CAD build for the part. Positions are in the model's coordinates, mm. Face numbers are marked on the shaded views. A direction names the side the tool comes from. Round coordinates to 2 decimals unless told otherwise and drop trailing zeros. Loops run counter-clockwise (first coordinate to the right, second up) from the corner with the lowest first, then second, coordinate; pieces in that order, holes last.
from build123d import *

# Parameters (mm, degrees)
BOSS_EXTRUDE1_DEPTH = 50
BOSS_EXTRUDE2_DEPTH = 5
SKETCH3_R           = 50
BOSS_EXTRUDE3_DEPTH = 5
FILLET1_R           = 5
BOSS_EXTRUDE4_START = 3
SKETCH5_R           = 50
BOSS_EXTRUDE4_DEPTH = 3
SKETCH5_3_R         = 4
CUT_EXTRUDE1_DEPTH  = 10


with BuildPart() as part:
    # Sketch1 → Boss-Extrude1 (new body)
    with BuildSketch(Plane(origin=(0, 0, 0), x_dir=(1, 0, 0), z_dir=(0, 1, 0))):
        Polygon((-14.60696181, 25.3), (-29.213923621, 0), (-14.60696181, -25.3), (14.60696181, -25.3), (29.213923621, 0), (14.60696181, 25.3), align=None)
        Polygon((-11.720210465, -20.3), (11.720210465, -20.3), (23.440420929, 0), (11.720210465, 20.3), (-11.720210465, 20.3), (-23.440420929, 0), align=None, mode=Mode.SUBTRACT)
    extrude(amount=BOSS_EXTRUDE1_DEPTH)

    # Sketch2 → Boss-Extrude2 (add)
    with BuildSketch(Plane(origin=(0, 50, 0), x_dir=(1, 0, 0), z_dir=(0, 1, 0))):
        Polygon((-14.60696181, 25.3), (-29.213923621, 0), (-14.60696181, -25.3), (14.60696181, -25.3), (29.213923621, 0), (14.60696181, 25.3), align=None)
    extrude(amount=BOSS_EXTRUDE2_DEPTH)

    # Sketch3 → Boss-Extrude3 (add)
    # profile 1 of 2: a face of its own
    with BuildSketch(Plane.XZ):
        with Locations(Location((0, 0, 0), (0, 0, 270))):
            Circle(SKETCH3_R)
        Polygon((-29.213923621, 0), (-14.60696181, -25.3), (14.60696181, -25.3), (29.213923621, 0), (14.60696181, 25.3), (-14.60696181, 25.3), align=None, mode=Mode.SUBTRACT)
    # profile 2 of 2: a face of its own
    with BuildSketch(Plane.XZ):
        Polygon((-14.60696181, 25.3), (-29.213923621, 0), (-14.60696181, -25.3), (14.60696181, -25.3), (29.213923621, 0), (14.60696181, 25.3), align=None)
        Polygon((-23.440420929, 0), (-11.720210465, 20.3), (11.720210465, 20.3), (23.440420929, 0), (11.720210465, -20.3), (-11.720210465, -20.3), align=None, mode=Mode.SUBTRACT)
    extrude(amount=-BOSS_EXTRUDE3_DEPTH)

    # Fillet1
    fillet1_edges = [part.edges().sort_by_distance(p)[0] for p in [
        (0, 5, -25.3),
        (-21.910442716, 5, 12.65),
        (-21.910442716, 5, -12.65),
        (21.910442716, 5, -12.65),
        (21.910442716, 5, 12.65),
        (0, 5, 25.3),
    ]]
    fillet(fillet1_edges, radius=FILLET1_R)

    # Sketch5 → Boss-Extrude4 (add)
    with BuildSketch(Plane.XZ.offset(BOSS_EXTRUDE4_START)):
        with Locations(Location((0, 0, 0), (0, 0, 270))):
            Circle(SKETCH5_R)
        Polygon((-4.252388339, -34.798222074), (3.484105268, -34.798222074), (7.352352072, -41.498222074), (3.484105268, -48.198222074), (-4.252388339, -48.198222074), (-8.120635142, -41.498222074), align=None, mode=Mode.SUBTRACT)
        Polygon((-32.262338492, -13.716434709), (-28.394091688, -20.416434709), (-32.262338492, -27.116434709), (-39.998832099, -27.116434709), (-43.867078902, -20.416434709), (-39.998832099, -13.716434709), align=None, mode=Mode.SUBTRACT)
        Polygon((28.009950153, -21.081787365), (31.878196957, -14.381787365), (39.614690564, -14.381787365), (43.482937367, -21.081787365), (39.614690564, -27.781787365), (31.878196957, -27.781787365), align=None, mode=Mode.SUBTRACT)
        Polygon((-28.009950153, 21.081787365), (-31.878196957, 14.381787365), (-39.614690564, 14.381787365), (-43.482937367, 21.081787365), (-39.614690564, 27.781787365), (-31.878196957, 27.781787365), align=None, mode=Mode.SUBTRACT)
        Polygon((-11.720210465, -20.3), (-23.440420929, 0), (-11.720210465, 20.3), (11.720210465, 20.3), (23.440420929, 0), (11.720210465, -20.3), align=None, mode=Mode.SUBTRACT)
        Polygon((32.262338492, 13.716434709), (28.394091688, 20.416434709), (32.262338492, 27.116434709), (39.998832099, 27.116434709), (43.867078902, 20.416434709), (39.998832099, 13.716434709), align=None, mode=Mode.SUBTRACT)
        Polygon((4.252388339, 34.798222074), (-3.484105268, 34.798222074), (-7.352352072, 41.498222074), (-3.484105268, 48.198222074), (4.252388339, 48.198222074), (8.120635142, 41.498222074), align=None, mode=Mode.SUBTRACT)
    extrude(amount=-BOSS_EXTRUDE4_DEPTH)

    # Sketch5_3 → Cut-Extrude1 (cut)
    with BuildSketch(Plane.XZ):
        with Locations(Location((0.384141535, 41.498222074, 0), (0, 0, 270))):
            Circle(SKETCH5_3_R)
        with Locations(Location((36.130585295, 20.416434709, 0), (0, 0, 270))):
            Circle(SKETCH5_3_R)
        with Locations(Location((35.74644376, -21.081787365, 0), (0, 0, 270))):
            Circle(SKETCH5_3_R)
        with Locations(Location((-0.384141535, -41.498222074, 0), (0, 0, 270))):
            Circle(SKETCH5_3_R)
        with Locations(Location((-36.130585295, -20.416434709, 0), (0, 0, 270))):
            Circle(SKETCH5_3_R)
        with Locations(Location((-35.74644376, 21.081787365, 0), (0, 0, 270))):
            Circle(SKETCH5_3_R)
    extrude(amount=-CUT_EXTRUDE1_DEPTH, mode=Mode.SUBTRACT)


solid = part.part
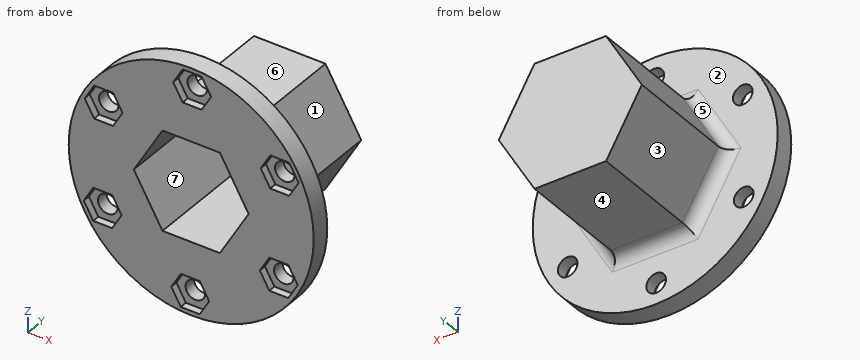
Item 1: Cut at A-A (y = 12). List the corners of the cut face in (x, z).
Verdict:
outline: (-29.21, 0) - (-14.61, -25.3) - (14.61, -25.3) - (29.21, 0) - (14.61, 25.3) - (-14.61, 25.3) - close; hole (-23.44, 0) - (-11.72, -20.3) - (11.72, -20.3) - (23.44, 0) - (11.72, 20.3) - (-11.72, 20.3) - close
Item 2: Wall check: L1, parallel to Z at x = -10.5, y = 43.5; L2, parallel to X at y = 1.5, z = -19; L3, parallel to Y at x = 10.5, z = 10. Give the ranges that are in metal, low to high.
Verdict:
L1: z = -25.3 to -20.3, 20.3 to 25.3
L2: x = -46.25 to -39.87, -32.39 to -12.47, 12.47 to 32.33, 39.16 to 46.25
L3: y = 50 to 55
Item 3: Flat gauge pins, fed straight in: P1, Ø6, axis at y = 47.5, z = 20, coming from the +X side; P2, Ø3.5, axis at x = -36.5, y = -2, coming from the +Z side; P3, Ø2.5, axis at x = 37, y = -1.5, coming from the -Z side; P4, Ø10.5, axis at x = -35, z = 18.5, coming from the -Y side. Where does each tip first touch, or does it go through?
Verdict:
P1: stops at x = 19.4
P2: stops at z = 35.95
P3: stops at z = -34.96
P4: stops at y = -3
Item 4: 3-axis set-ups, long thin cutter, end or side, ignore diameter. For the marked faces 1, 2, 3 and 4: which of +Z, -Z, +X, -X, +Y, -Y reach the whole face in a straight line?
Verdict:
face 1: +Z, +X, +Y
face 2: +Y
face 3: -Z, -X, +Y
face 4: -Z, +X, -X, +Y
Item 5: Mould opens along X. For the marked faces 5, 6 and 7 say: released by +X, released by -X, zero draft, split by the parting line, or undercut.
Verdict:
face 5: released by -X
face 6: zero draft
face 7: undercut
Item 6: Cut at B-B (z = 43.5). List the corners of the cut face in (x, y), plus the area to 3 significant figures.
Verdict:
outline: (-24.65, -3) - (-6.2, -3) - (-6.2, 0) - (-3.08, 0) - (-3.08, 5) - (-24.65, 5) - close; (3.85, 0) - (6.96, 0) - (6.96, -3) - (24.65, -3) - (24.65, 5) - (3.85, 5) - close
area: 320 mm2
Item 7: Cut at C-C (x = 13). List the corners of the cut face in (y, z), plus the area to 3 significant figures.
Verdict:
outline: (-3, -48.28) - (5, -48.28) - (5, -30.3) arc R5 cw to (10, -25.3) - (55, -25.3) - (55, 25.3) - (10, 25.3) arc R5 cw to (5, 30.3) - (5, 48.28) - (-3, 48.28) - (-3, 18.08) - (50, 18.08) - (50, -18.08) - (-3, -18.08) - close
area: 1,400 mm2
